from build123d import *

# Parameters (mm, degrees)
SKETCH_1_R      = 1.75
SKETCH_1_R_2    = 1.3
EXTRUDE_1_DEPTH = 3


with BuildPart() as part:
    # Sketch 1 → Extrude 1 (new body)
    with BuildSketch(Plane(origin=(0, 0, 0), x_dir=(1, 0, 0), z_dir=(0, 1, 0))):
        with BuildLine():
            Line((-73, 57), (73, 57))
            ThreePointArc((73, 57), (75.121320344, 56.121320344), (76, 54))
            Line((76, 54), (76, -54))
            ThreePointArc((76, -54), (75.121320344, -56.121320344), (73, -57))
            Line((73, -57), (-73, -57))
            ThreePointArc((-73, -57), (-75.121320344, -56.121320344), (-76, -54))
            Line((-76, -54), (-76, 54))
            ThreePointArc((-76, 54), (-75.121320344, 56.121320344), (-73, 57))
        make_face()
        with Locations(Location((-71, 52, 0), (0, 0, 270))):
            Circle(SKETCH_1_R, mode=Mode.SUBTRACT)
        with Locations(Location((71, 52, 0), (0, 0, 270))):
            Circle(SKETCH_1_R, mode=Mode.SUBTRACT)
        with Locations(Location((71, -52, 0), (0, 0, 270))):
            Circle(SKETCH_1_R, mode=Mode.SUBTRACT)
        with Locations(Location((-71, -52, 0), (0, 0, 270))):
            Circle(SKETCH_1_R, mode=Mode.SUBTRACT)
        with Locations(Location((-56, 43, 0), (0, 0, 270))):
            Circle(SKETCH_1_R_2, mode=Mode.SUBTRACT)
        with Locations(Location((-56, -43, 0), (0, 0, 270))):
            Circle(SKETCH_1_R_2, mode=Mode.SUBTRACT)
        with Locations(Location((56, -43, 0), (0, 0, 90))):
            Circle(SKETCH_1_R_2, mode=Mode.SUBTRACT)
        with Locations(Location((56, 43, 0), (0, 0, 90))):
            Circle(SKETCH_1_R_2, mode=Mode.SUBTRACT)
        with BuildLine():
            Line((-2, 44.3), (2, 44.3))
            ThreePointArc((2, 44.3), (3.3, 43), (2, 41.7))
            Line((2, 41.7), (-2, 41.7))
            ThreePointArc((-2, 41.7), (-3.3, 43), (-2, 44.3))
        make_face(mode=Mode.SUBTRACT)
        with BuildLine():
            Line((-2, -41.7), (2, -41.7))
            ThreePointArc((2, -41.7), (3.3, -43), (2, -44.3))
            Line((2, -44.3), (-2, -44.3))
            ThreePointArc((-2, -44.3), (-3.3, -43), (-2, -41.7))
        make_face(mode=Mode.SUBTRACT)
    extrude(amount=EXTRUDE_1_DEPTH)


solid = part.part
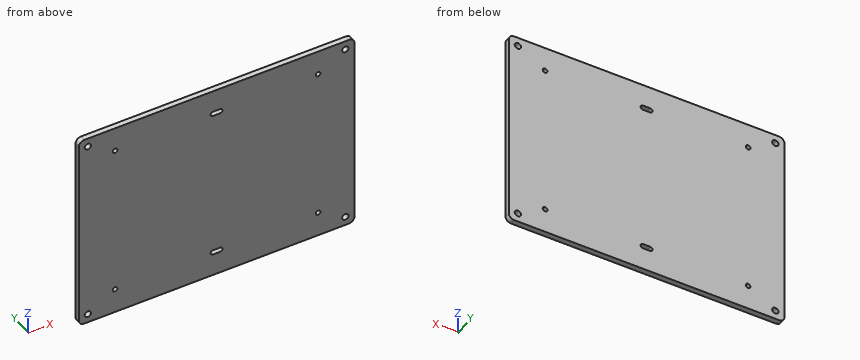
The listing builds one solid part. Answer for the finished solid, in the listing's coordinates (mm). Coordinates: 2 decimals unless noted, no trailing zeros. Loops run counter-clockwise (first coordinate to the right, second up) from the corner with the lowest first, then second, coordinate; pieces in that order, holes last. Notation, with made-up numbers: (36, -13) -> (48, -13) arc R23 ccw to (48, 26) -> close; hole circle Ø5 at (81.5, 38.5). An arc over 180 degrees is marked (long way). Write item = value, one per line. Start each with the question number.
1) Straight lines are drawn through the part: line 1 (X direction, y = 1.7, z = 43); line 2 (Z direction, x = 56, y = 2.3); line 3 (X direction, y = 2.1, z = 52). For each, find the intervals that lie inside material, in ascending order. Write a range as from..to.
2) A cutting plane is placed at A-A (z = 52). Give the vertices of the cut face in (x, y), then the cut area to 3 significant figures.
3) Given pin 1 Ø3 at (x, z) = (-56, -43) entering from +Y; pin 2 Ø3 at (x, z) = (-71, 52) entering from -Y, each flat-ended and moving along its own axis, determine where each tip first touches the part or whether it passes through.
4) A cutting plane is placed at B-B (x = 71). Give the vertices of the cut face in (y, z), then the cut area to 3 significant figures.
Responses:
q1.line_1 = -76..-57.3, -54.7..-3.3, 3.3..54.7, 57.3..76
q1.line_2 = -57..-44.3, -41.7..41.7, 44.3..57
q1.line_3 = -76..-72.75, -69.25..69.25, 72.75..76
q2.outline = (-76, 0) -> (-72.75, 0) -> (-72.75, 3) -> (-76, 3) -> close; (-69.25, 0) -> (69.25, 0) -> (69.25, 3) -> (-69.25, 3) -> close; (72.75, 0) -> (76, 0) -> (76, 3) -> (72.75, 3) -> close
q2.area = 435 mm²
q3.pin_1 = 3
q3.pin_2 = through
q4.outline = (0, -57) -> (3, -57) -> (3, -53.75) -> (0, -53.75) -> close; (0, -50.25) -> (3, -50.25) -> (3, 50.25) -> (0, 50.25) -> close; (0, 53.75) -> (3, 53.75) -> (3, 57) -> (0, 57) -> close
q4.area = 321 mm²
